from build123d import *

# Parameters (mm, degrees)
F0_W     = 457.2
F0_H     = 254
F1_DEPTH = 12.7
F2_W     = 19.05
F2_H     = 228.6
F3_DEPTH = 165.1
F4_W     = 19.05
F4_H     = 63.5
F5_DEPTH = 419.1
F6_W     = 419.1
F6_H     = 19.05
F7_DEPTH = 165.1
F8_W     = 165.1
F8_H     = 19.05
F9_DEPTH = 419.1


with BuildPart() as f1:
    # F0 (on Front) → F1 (new body)
    with BuildSketch(Plane.XZ):
        Rectangle(F0_W, F0_H)
    extrude(amount=F1_DEPTH)

    # F2 (on face) → F3 (join)
    with BuildSketch(Plane.XZ.offset(12.7)):
        with Locations((-219.075, -12.7)):
            Rectangle(F2_W, F2_H)
        with Locations((219.075, -12.7)):
            Rectangle(F2_W, F2_H)
    extrude(amount=F3_DEPTH)

    # F4 (on face) → F5 (join, through all)
    with BuildSketch(Plane.YZ.offset(-209.55)):
        with Locations((-168.275, 57.15)):
            Rectangle(F4_W, F4_H)
    extrude(amount=F5_DEPTH)

    # F6 (on face) → F7 (join, through all)
    with BuildSketch(Plane.XZ.offset(12.7)):
        with Locations((0, 15.875)):
            Rectangle(F6_W, F6_H)
    extrude(amount=F7_DEPTH)

    # F8 (on face) → F9 (join, through all)
    with BuildSketch(Plane.YZ.offset(-209.55)):
        with Locations((-95.25, -79.375)):
            Rectangle(F8_W, F8_H)
    extrude(amount=F9_DEPTH)


solid = f1.part
Build history of the part. All positions in model axes, mm. A direction names the side the tool comes from. Coordinates: 2 decimals unless noted, no trailing zeros. Write each loop counter-clockwise with the first axis right and the second up, starting at its lowest first coordinate (ties: lowest second). Pieces come first, ordered by that corner, then holes.
(1) 3-axis set-ups, long thin cutter, end or side, ignore diameter. For faces 4 (the flat face through (-3, -12.7, -31)), 5 (the flat face through (209.55, -94, 63)), 6 (the flat face through (219, -94, 101.6)), 7 (the flat face through (-3, -96, -88.9)): which of +Z, -Z, +X, -X, +Y, -Y reach the whole face in a straight line?
(2) Mould opens along Z. For faces 1 (the flat face through (-3, -12.7, 77)), 2 (the flat face through (-3, -94, 6.35)), 3 (the flat face through (-3, -85, 25.4)) say: pulls with the +Z half, pulls with the -Z half, needs draft (parallel to the pull), parting line crosses it, or undercut.
(3) Drill centre lines: line 1 (Z direction, x = -41, y = -134); line 2 (X direction, y = -152.5, z = -43); line 3 (Z direction, x = -106.5, y = -163). Where is each one in solid material? Low to high.
(4) Cut at A-A on z = 36. List the corners of the cut face in (x, y), and give its area (3 significant figures).
(5) Pin check, flat tips, straight feed: pin 1 Ø2 at (x, y) = (113.5, -89.5) entering from +Z; pin 2 Ø5.5 at (x, y) = (-217.5, -71.5) entering from +Z; pin 3 Ø3 at (x, z) = (-30, 19.5) entering from +Y; pin 4 Ø5.5 at (x, y) = (64.5, -167) entering from +Z. Stop position of each tip, or through.
(6) Cut at D-D on z = -102. List the corners of the cut face in (x, y).
(7) Cut at C-C on x = 134. List the corners of the cut face in (y, z), and give its area (3 significant figures).
(8) Cut at B-B on y = -114. List the corners of the cut face in (x, z).
Working result:
1. face 4: -Y
1. face 5: +Z
1. face 6: +Z, +X, -X, -Y
1. face 7: -Z, -Y
2. face 1: needs draft
2. face 2: undercut
2. face 3: pulls with the +Z half
3. line 1: z = -88.9 to -69.85, 6.35 to 25.4
3. line 2: x = -228.6 to -209.55, 209.55 to 228.6
3. line 3: z = -88.9 to -69.85, 6.35 to 88.9
4. outline: (-228.6, -177.8) - (228.6, -177.8) - (228.6, 0) - (-228.6, 0) - close; hole (-209.55, -158.75) - (209.55, -158.75) - (209.55, -12.7) - (-209.55, -12.7) - close
4. area: 20,100 mm2
5. pin 1: stops at z = 25.4
5. pin 2: stops at z = 101.6
5. pin 3: stops at y = 0
5. pin 4: stops at z = 88.9
6. outline: (-228.6, -177.8) - (-209.55, -177.8) - (-209.55, -12.7) - (209.55, -12.7) - (209.55, -177.8) - (228.6, -177.8) - (228.6, 0) - (-228.6, 0) - close
7. outline: (-177.8, -88.9) - (-12.7, -88.9) - (-12.7, -127) - (0, -127) - (0, 127) - (-12.7, 127) - (-12.7, 25.4) - (-158.75, 25.4) - (-158.75, 88.9) - (-177.8, 88.9) - (-177.8, 6.35) - (-12.7, 6.35) - (-12.7, -69.85) - (-177.8, -69.85) - close
7. area: 10,700 mm2
8. outline: (-228.6, -127) - (-209.55, -127) - (-209.55, -88.9) - (209.55, -88.9) - (209.55, -127) - (228.6, -127) - (228.6, 101.6) - (209.55, 101.6) - (209.55, 25.4) - (-209.55, 25.4) - (-209.55, 101.6) - (-228.6, 101.6) - close; hole (-209.55, -69.85) - (209.55, -69.85) - (209.55, 6.35) - (-209.55, 6.35) - close
